from build123d import *

# Parameters (mm, degrees)
F0_W     = 372.93318
F0_H     = 239.700406
F1_DEPTH = 25.4
F3_D     = 19.05


with BuildPart() as f1:
    # F0 (on Front) → F1 (new body)
    with BuildSketch(Plane.XZ):
        Rectangle(F0_W, F0_H)
    extrude(amount=F1_DEPTH)

    # F3 (through all)
    with Locations(Plane.XZ.offset(25.4)):
        with Locations((-135.66659, 81.750203), (-135.66659, -70.649797), (118.33341, -70.649797)):
            Hole(F3_D / 2)


solid = f1.part
Can you work these out from the model? Positions are in its coordinate system, mm. Coordinates: 2 decimals unless noted, no trailing zeros. Order: outer loops, then holes, each group sorted by start corner. A loop starts at its lowest first (then second) coordinate and runs counter-clockwise, first axis right, second up. Notation, with made-up numbers: M -3,-24.75 L 27,-24.75 A19 cw 27,-2.75 Z; hole C 66,84.5 d2. An arc over 180 degrees is marked long. Write item = value, one per line.
(1) I need wall thicknesses on line 1 along X through (y, z) = (-12.75, -75); line 2 along Z through (x, y) = (-128, -11.25); line 3 along X through (y, z) = (-4.5, 90.5). Which ranges of each line are inside material? Lowest first, please. Write a range as [from, to].
Results are:
line_1 = [-186.47, -144.14], [-127.19, 109.86], [126.81, 186.47]
line_2 = [-119.85, -76.3], [-65, 76.1], [87.4, 119.85]
line_3 = [-186.47, -139.43], [-131.9, 186.47]
(2) Suppose I cut it at B-B on z = 78. Please give me the cut outline in (x, y).
Results are:
outline = M -186.47,-25.4 L -144.42,-25.4 L -144.42,0 L -186.47,0 Z; M -126.91,-25.4 L 186.47,-25.4 L 186.47,0 L -126.91,0 Z
(3) If we mould it in two halves opening along X, with no side actions, what happens to faces 1 (the face through (-186.467, -13, -2)), 2 (the face through (-3, 0, 2)), 3 (the face through (186.467, -13, -2)), 4 (the face through (-133.602, -12.522, 72.452))? For each: pulls with the +X half, pulls with the -X half, needs draft (parallel to the pull), parting line crosses it, or undercut.
Results are:
face_1 = pulls with the -X half
face_2 = needs draft
face_3 = pulls with the +X half
face_4 = undercut
(4) For pin 1 Ø6 at (x, z) = (92, -33.5) entering from +Y; pin 2 Ø11.5 at (x, z) = (-135.67, -70.65) entering from -Y, each with a flat end and sliding along its axis, tell me the tip position at first contact or that it passes through.
Results are:
pin_1 = 0
pin_2 = through
(5) Suppose I cut it at A-A on z = -75. Please give me the cut outline in (x, y).
Results are:
outline = M -186.47,-25.4 L -144.14,-25.4 L -144.14,0 L -186.47,0 Z; M -127.19,-25.4 L 109.86,-25.4 L 109.86,0 L -127.19,0 Z; M 126.81,-25.4 L 186.47,-25.4 L 186.47,0 L 126.81,0 Z
